Can you work these out from the model? Positions are in its coordinate system, mm. A direction names the side the tool comes from. Give positions to 0.01 mm unless a question says otherwise; leave off trailing zeros. Order: outer loops, then holes, each group sorted by start corner. A loop starts at its lowest first (then second) coordinate and runs counter-clockwise, first axis right, second up. Notation, with made-up numbers: M -38.75,-3.75 L 14.25,-3.75 A22 cw 14.25,11.25 Z; hole C -14.5,12.5 d8. An arc over 180 degrees is marked long. One line per question, with ' | ' between items. Start each with the question number.
1) If we section it at B-B, the plane x = 15: Please give me the cut outline in (y, z), plus the area to 3 significant figures.
2) Please list where these lines run through material, in increasing order: line 1 along Z through (x, y) = (28.5, 0.8); line 2 along X through (y, z) = (1.5, -21.5); line 3 along Z through (x, y) = (3.5, 7). Write a range as [from, to].
3) If we section it at D-D, the plane x = -28.5: Please give me the cut outline in (y, z), plus the area to 3 significant figures.
4) Thinking about a two-plate mould opening in X: for faces 4 (the flat face through (0, 12, -22.5)), 5 (the flat face through (29, 1, 18)), 6 (the flat face through (32, 1, 21)), which applies, +X half, -X half, draft (parallel to the pull), parting line (faces both ways), or undercut?
5) I'm going to push flat-ended pins straight in: pin 1 Ø10 at (y, z) = (14.5, -0.5) entering from -X; pin 2 Ø4 at (x, z) = (28.5, -21.5) entering from +Y; pin 3 Ø1.5 at (y, z) = (4.5, -10.5) entering from +X; pin 4 Ø2 at (x, z) = (-28.5, 21.5) entering from +Y. Where does each tip first touch, or does it pass through?
6) If we section it at A-A, the plane z = 12: Please give me the cut outline in (x, y), plus the area to 3 significant figures.
7) For faces 1 (the flat face through (0, 12, 22.5)), 2 (the flat face through (-30, 2.5, -23)), 3 (the flat face through (30, 2.5, 23)), which set-ups out of +Z, -Z, +X, -X, +Y, -Y let a thin tool reach every point of the face, with its end or its side?
8) If we section it at C-C, the plane y = 1.5: Please give me the cut outline in (x, z).
```python
from build123d import *

# Parameters (mm, degrees)
SKIZZE1_W                       = 50
SKIZZE1_H                       = 50
SKIZZE1_W_2                     = 45
SKIZZE1_H_2                     = 45
AUFSATZ_LINEAR_AUSTRAGEN1_DEPTH = 25
SKIZZE2_W                       = 7
SKIZZE2_H                       = 7
SKIZZE2_R                       = 1.8
AUFSATZ_LINEAR_AUSTRAGEN2_DEPTH = 2.5
SPIEGELN2_COPY_1_SKETCH_W       = 7
SPIEGELN2_COPY_1_SKETCH_H       = 7
SPIEGELN2_COPY_1_SKETCH_R       = 1.8
SPIEGELN2_COPY_1_DEPTH          = 2.5


with BuildPart() as part:
    # Skizze1 → Aufsatz-Linear austragen1 (new body)
    with BuildSketch(Plane(origin=(0, 0, 0), x_dir=(1, 0, 0), z_dir=(0, 1, 0))):
        Rectangle(SKIZZE1_W, SKIZZE1_H)
        Rectangle(SKIZZE1_W_2, SKIZZE1_H_2, mode=Mode.SUBTRACT)
    extrude(amount=AUFSATZ_LINEAR_AUSTRAGEN1_DEPTH)

    # Skizze2 → Aufsatz-Linear austragen2 (add)
    with BuildSketch(Plane.XZ):
        with Locations((-28.5, 21.5)):
            Rectangle(SKIZZE2_W, SKIZZE2_H)
        with Locations((-28.5, 21.5)):
            Circle(SKIZZE2_R, mode=Mode.SUBTRACT)
    aufsatz_linear_austragen2 = extrude(amount=-AUFSATZ_LINEAR_AUSTRAGEN2_DEPTH)

    # Spiegeln1: Aufsatz-Linear austragen2 across plane
    add(aufsatz_linear_austragen2.mirror(Plane(origin=(0, 0, 0), x_dir=(0, 0, 1), z_dir=(1, 0, 0))))

    # Spiegeln2: Aufsatz-Linear austragen2 across plane
    add(aufsatz_linear_austragen2.mirror(Plane.XY))

    # Spiegeln2 copy 1 sketch → Spiegeln2 copy 1 (add)
    with BuildSketch(Plane(origin=(0, 0, 0), x_dir=(-1, 0, 0), z_dir=(0, -1, 0))):
        with Locations((-28.5, 21.5)):
            Rectangle(SPIEGELN2_COPY_1_SKETCH_W, SPIEGELN2_COPY_1_SKETCH_H)
        with Locations((-28.5, 21.5)):
            Circle(SPIEGELN2_COPY_1_SKETCH_R, mode=Mode.SUBTRACT)
    extrude(amount=-SPIEGELN2_COPY_1_DEPTH)


solid = part.part
```
Results found:
1) outline: M 0,-25 L 25,-25 L 25,-22.5 L 0,-22.5 Z; M 0,22.5 L 25,22.5 L 25,25 L 0,25 Z | area: 125 mm²
2) line 1: z = [-25, -23.3], [-19.7, -18], [18, 19.7], [23.3, 25] | line 2: x = [-32, -30.3], [-26.7, -22.5], [22.5, 26.7], [30.3, 32] | line 3: z = [-25, -22.5], [22.5, 25]
3) outline: M 0,-25 L 2.5,-25 L 2.5,-23.3 L 0,-23.3 Z; M 0,-19.7 L 2.5,-19.7 L 2.5,-18 L 0,-18 Z; M 0,18 L 2.5,18 L 2.5,19.7 L 0,19.7 Z; M 0,23.3 L 2.5,23.3 L 2.5,25 L 0,25 Z | area: 17.0 mm²
4) face 4: undercut | face 5: draft | face 6: +X half
5) pin 1: stops at x = -25 | pin 2: stops at y = 2.5 | pin 3: stops at x = 25 | pin 4: passes through
6) outline: M -25,0 L -22.5,0 L -22.5,25 L -25,25 Z; M 22.5,0 L 25,0 L 25,25 L 22.5,25 Z | area: 125 mm²
7) face 1: +Y, -Y | face 2: +Z, -Z, -X, +Y | face 3: +Z, -Z, +X, +Y
8) outline: M -32,-25 L 32,-25 L 32,-18 L 25,-18 L 25,18 L 32,18 L 32,25 L -32,25 L -32,18 L -25,18 L -25,-18 L -32,-18 Z; hole C -28.5,-21.5 d3.6; hole C -28.5,21.5 d3.6; hole M -22.5,-22.5 L 22.5,-22.5 L 22.5,22.5 L -22.5,22.5 Z; hole C 28.5,-21.5 d3.6; hole C 28.5,21.5 d3.6
